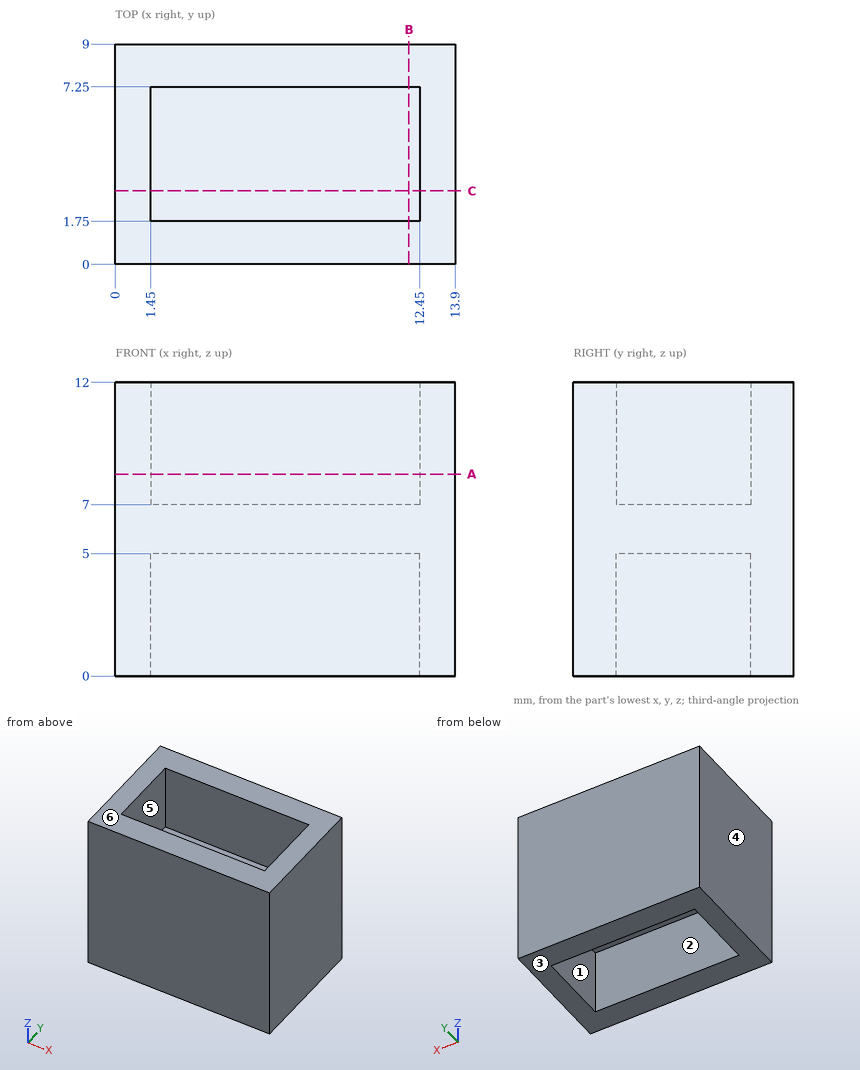
Drawing for the job (mm, zero at the part's lowest x, y, z). A direction names the side the tool comes from. Round coordinates to 2 decimals unless told otherwise and drop trailing zeros. Write each loop counter-clockwise with the first axis right and the second up, starting at its lowest first coordinate (ties: lowest second). Pieces come first, ordered by that corner, then holes. Notation, with made-up numbers: (40, 77) - (57, 77) arc R14 cw to (57, 91) - close; hole circle Ø4 at (57, -26). An arc over 180 degrees is marked (long way). Return JSON: item names as keys, results as strings. Group by question number.
Item 1: Band-saw the part on A-A on z = 8.25. List the corners of the cut face in (x, y).
Item 2: Probe probe 1 along Y at (x, z) = (10, 8.5); probe 2 along X at (y, z) = (3.25, 11.25); probe 3 along Z at (x, y) = (1.5, 3.75). List the from-to ranges inside material, lowest first.
Item 3: Band-saw the part on B-B on x = 12. List the corners of the cut face in (y, z), plus the area to 3 significant figures.
Item 4: 3-axis set-ups, long thin cutter, end or side, ignore diameter. For the marked faces 5 and 6: which of +Z, -Z, +X, -X, +Y, -Y reach the whole face in a straight line?
Item 5: Flat gauge pins, fed straight in: pin 1 Ø4.5 at (x, y) = (5, 4.5) entering from -Z; pin 2 Ø1.5 at (y, z) = (4.5, 9) entering from -X; pin 3 Ø3 at (x, y) = (10, 3.5) entering from +Z. Where does each tip first touch, or does it go through?
Item 6: Band-saw the part on C-C on y = 3. List the corners of the cut face in (x, z).
Item 7: Mould opens along X. For the marked faces 1, 2, 3 and 4 say: +X half, -X half, draft (parallel to the pull), parting line (faces both ways), or undercut.
Resolved:
{
 "1": {"outline": "(0, 0) - (13.9, 0) - (13.9, 9) - (0, 9) - close; hole (1.45, 1.75) - (12.45, 1.75) - (12.45, 7.25) - (1.45, 7.25) - close"},
 "2": {"probe 1": "y = 0 to 1.75, 7.25 to 9", "probe 2": "x = 0 to 1.45, 12.45 to 13.9", "probe 3": "z = 5 to 7"},
 "3": {"outline": "(0, 0) - (1.75, 0) - (1.75, 5) - (7.25, 5) - (7.25, 0) - (9, 0) - (9, 12) - (7.25, 12) - (7.25, 7) - (1.75, 7) - (1.75, 12) - (0, 12) - close", "area": "53.0 mm²"},
 "4": {"face 5": "+Z", "face 6": "+Z, +X, -X, +Y, -Y"},
 "5": {"pin 1": "stops at z = 5", "pin 2": "stops at x = 0", "pin 3": "stops at z = 7"},
 "6": {"outline": "(0, 0) - (1.45, 0) - (1.45, 5) - (12.45, 5) - (12.45, 0) - (13.9, 0) - (13.9, 12) - (12.45, 12) - (12.45, 7) - (1.45, 7) - (1.45, 12) - (0, 12) - close"},
 "7": {"face 1": "undercut", "face 2": "undercut", "face 3": "draft", "face 4": "-X half"}
}
